Could you check a few things on this model? Use its own coordinates, in mm. A direction names the side the tool comes from. Round coordinates to 2 decimals unless told otherwise and drop trailing zeros. Loops run counter-clockwise (first coordinate to the right, second up) from the corner with the lowest first, then second, coordinate; pieces in that order, holes last. Notation, with made-up numbers: (55.5, -7.5) -> (79.5, -7.5) arc R8 cw to (79.5, 5.5) -> close; hole circle Ø9 at (22.5, -17.5). An arc over 180 degrees is marked (long way). One line per item, written item: value.
from build123d import *

# Parameters (mm, degrees)
SKETCH_1_W          = 120
SKETCH_1_H          = 40
EXTRUDE_1_DEPTH     = 20
SKETCH_2_W          = 18
SKETCH_2_H          = 40
CUT_EXTRUDE_1_DEPTH = 3
CHAMFER_1_SIZE      = 5


with BuildPart() as part:
    # 草图1 → 凸台-拉伸1 (new, symmetric)
    with BuildSketch(Plane.XY):
        Rectangle(SKETCH_1_W, SKETCH_1_H)
    extrude(amount=EXTRUDE_1_DEPTH, both=True)

    # 草图2 → 切除-拉伸1 (cut)
    with BuildSketch(Plane.XY.offset(20)):
        Rectangle(SKETCH_2_W, SKETCH_2_H)
    extrude(amount=-CUT_EXTRUDE_1_DEPTH, mode=Mode.SUBTRACT)

    # 倒角1
    chamfer_1_edges = [part.edges().sort_by_distance(p)[0] for p in [
        (60, -20, 0),
        (-60, -20, 0),
        (-60, 20, 0),
        (60, 20, 0),
    ]]
    chamfer(chamfer_1_edges, length=CHAMFER_1_SIZE)


solid = part.part
(1) If I drill on L1, parallel to Z at x = 5.5, y = 8.5; L2, parallel to X at y = -17.5, z = 9.5; L3, parallel to X at y = 16.5, z = -13, over which ranges is the centre line in solid material (lowest first)?
Recorded:
L1: -20 to 17
L2: -57.5 to 57.5
L3: -58.5 to 58.5
(2) If we section it at A-A, the plane y = -16.5: Please give me the cut outline in (x, z).
Recorded:
outline: (-58.5, -20) -> (58.5, -20) -> (58.5, 20) -> (9, 20) -> (9, 17) -> (-9, 17) -> (-9, 20) -> (-58.5, 20) -> close
(3) If we section it at B-B, the plane x = -4.5: Please give me the cut outline in (y, z).
Recorded:
outline: (-20, -20) -> (20, -20) -> (20, 17) -> (-20, 17) -> close
(4) For faces 4 (the face through (0, 0, 17)), 5 (the face through (-1, 0, -20)), which set-ups out of +Z, -Z, +X, -X, +Y, -Y let a thin tool reach every point of the face, with its end or its side?
Recorded:
face 4: +Z, +Y, -Y
face 5: -Z, +X, -X, +Y, -Y
(5) I'm going to push a flat-ended pin straight in: pin 1 Ø1 at (x, y) = (5.5, 10) entering from +Z. Where does the tip first touch, or does it pass through?
Recorded:
pin 1: z = 17
(6) Thinking about a two-plate mould opening in X: for faces 1 (the face through (-9, 0, 19)), 2 (the face through (60, 0, 0)), 3 (the face through (-35, 0, 20)), which applies, released by +X, released by -X, zero draft, split by the parting line, or undercut?
Recorded:
face 1: undercut
face 2: released by +X
face 3: zero draft
